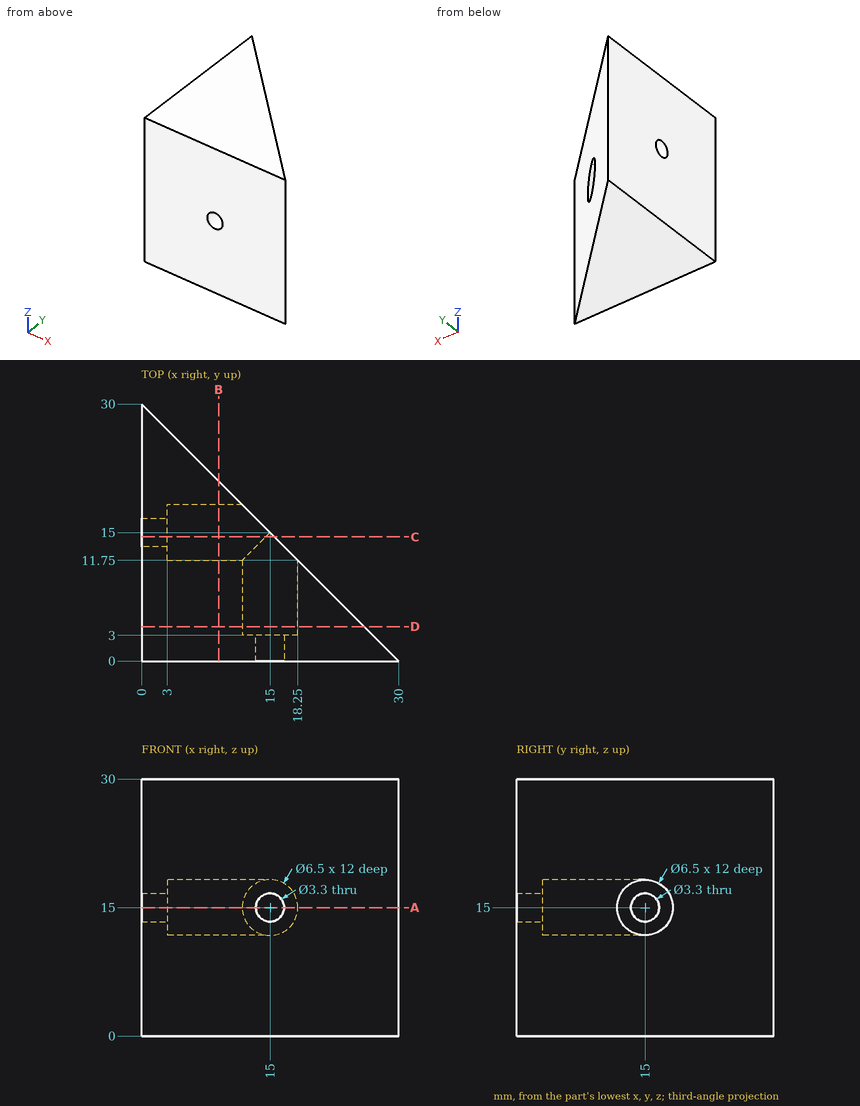
Verification items for this drawing (mm, ordinates from the low corner). Coordinates: 2 decimals unless noted, no trailing zeros. Write each loop counter-clockwise with the first axis right and the second up, starting at its lowest first coordinate (ties: lowest second). Pieces come first, ordered by that corner, then holes. Notation, with made-up numbers: M 14.5,-27 L 39.5,-27 A6 ccw 39.5,-23 Z; hole C 44.5,17 d8. An arc over 180 degrees is marked long. Use one line per item in the form item = value. Start each with the question number.
1) Section check A-A on z = 15. Enter the section's corners in (x, y), and give its area (3 significant figures).
2) Thickness scan on probe 1 along Z at (x, y) = (0.95, 15); probe 2 along Z at (x, y) = (15, 8); probe 3 along X at (y, z) = (15, 9). Record the ranges inside material, lowest first. Write a range as from..to.
3) Section check B-B on x = 9. Enter the section's corners in (y, z).
4) Go/stop test with flat-tipped pins: pin 1 Ø5 at (y, z) = (15, 15) entering from -X; pin 2 Ø2 at (y, z) = (15.5, 16.5) entering from +X; pin 3 Ø10.5 at (x, z) = (15, 15) entering from +Y; pin 4 Ø5.5 at (x, z) = (15, 15) entering from +Y. Record where each tip stops, or that it passes through.
5) Section check C-C on y = 14.5. Enter the section's corners in (x, z), and give its area (3 significant figures).
6) Section check D-D on y = 4. Enter the section's corners in (x, z), and give its area (3 significant figures).
Responses:
q1.outline = M 0,0 L 13.35,0 L 13.35,3 L 11.75,3 L 11.75,11.75 L 3,11.75 L 3,13.35 L 0,13.35 Z; M 0,16.65 L 3,16.65 L 3,18.25 L 11.75,18.25 L 0,30 Z; M 16.65,0 L 30,0 L 18.25,11.75 L 18.25,3 L 16.65,3 Z
q1.area = 295 mm2
q2.probe_1 = 0..13.35, 16.65..30
q2.probe_2 = 0..11.75, 18.25..30
q2.probe_3 = 0..15
q3.outline = M 0,0 L 21,0 L 21,30 L 0,30 Z; hole C 15,15 d6.5
q4.pin_1 = 0
q4.pin_2 = 3
q4.pin_3 = 20.25
q4.pin_4 = 3
q5.outline = M 0,0 L 15.5,0 L 15.5,11.79 A3.25 cw 14.5,11.79 L 3,11.79 L 3,13.43 L 0,13.43 Z; M 0,16.57 L 3,16.57 L 3,18.21 L 14.5,18.21 A3.25 cw 15.5,18.21 L 15.5,30 L 0,30 Z
q5.area = 375 mm2
q6.outline = M 0,0 L 26,0 L 26,30 L 0,30 Z; hole C 15,15 d6.5
q6.area = 747 mm2
